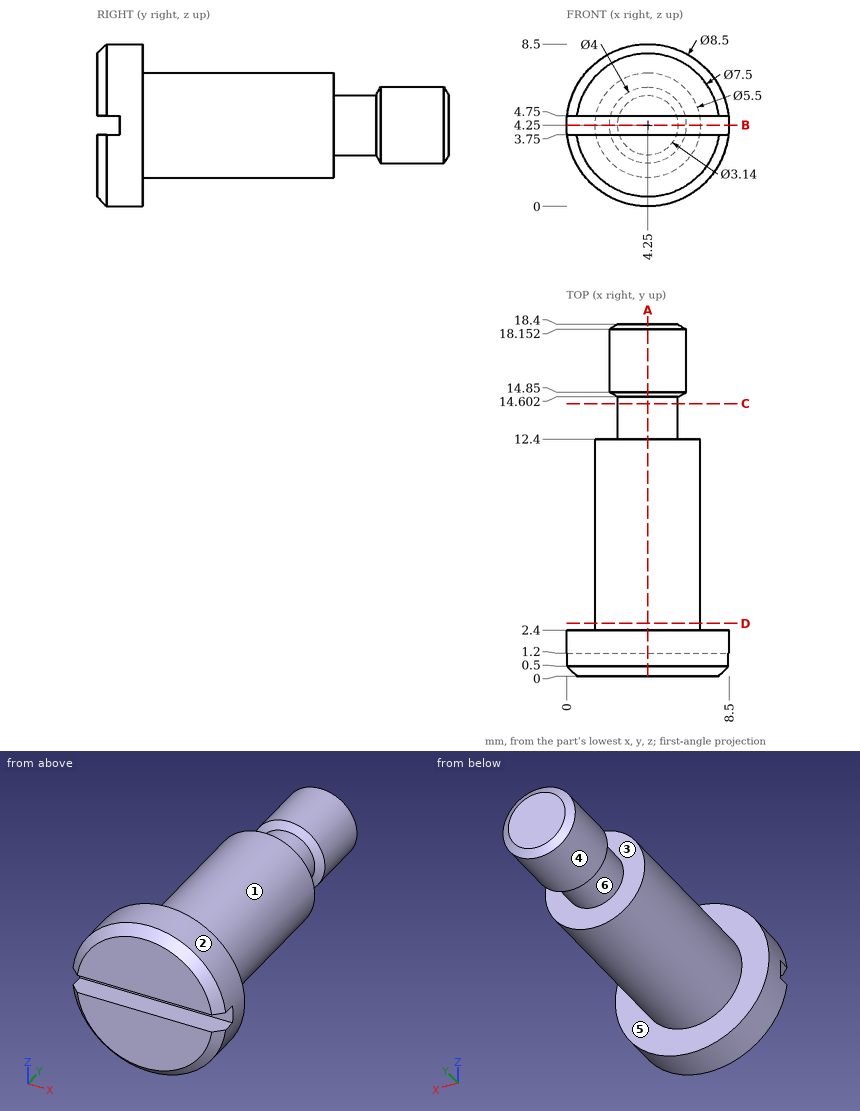
Verification items for this drawing (mm, ordinates from the low corner). A direction names the side the tool comes from. Round coordinates to 2 decimals unless told otherwise and drop trailing zeros. Loops run counter-clockwise (first coordinate to the right, second up) from the corner with the lowest first, then second, coordinate; pieces in that order, holes last. Notation, with made-up numbers: (-19, 29) -> (23, 29) arc R18 cw to (23, 38) -> close; hole circle Ø4 at (25, 33.5). An arc over 180 degrees is marked (long way). Answer in a Markdown table with one row per item.
Q1. Thickness scan on L1, parallel to Y at x = 1.75, z = 1.75; L2, parallel to Y at x = 4, z = 2; L3, parallel to Z at x = 5.25, y = 10.75. Record the ranges inside material, lowest first.
Data:
| item | result |
|---|---|
| L1 | y = 0 to 2.4 |
| L2 | y = 0 to 12.4 |
| L3 | z = 1.69 to 6.81 |
Q2. Sectioned sample at C-C on y = 14.25. Enter the section's corners in (x, z).
Data:
| item | result |
|---|---|
| outline | circle Ø3.14 at (4.25, 4.25) |
Q3. Go/stop test with flat-tipped pins: P1, Ø3, axis at x = 7, y = 14.5, coming from the -Z side; P2, Ø4, axis at x = 2.5, y = 5.5, coming from the +Z side; P3, Ø3, axis at x = 6.5, y = 14.5, coming from the +Z side. Record where each tip stops, or that it passes through.
Data:
| item | result |
|---|---|
| P1 | stops at z = 2.72 |
| P2 | stops at z = 7 |
| P3 | stops at z = 6.09 |
Q4. Sectioned sample at B-B on z = 4.25. Enter the section's corners in (x, y), then the cut area to 3 significant figures.
Data:
| item | result |
|---|---|
| outline | (0, 1.2) -> (8.5, 1.2) -> (8.5, 2.4) -> (7, 2.4) -> (7, 12.4) -> (5.82, 12.4) -> (5.82, 14.6) -> (6.25, 14.85) -> (6.25, 18.15) -> (5.82, 18.4) -> (2.68, 18.4) -> (2.25, 18.15) -> (2.25, 14.85) -> (2.68, 14.6) -> (2.68, 12.4) -> (1.5, 12.4) -> (1.5, 2.4) -> (0, 2.4) -> close |
| area | 87.1 mm^2 |
Q5. Release check for a two-part mould opening along Y. For the marked faces 3, 4, 5 and 6 record: released by +Y, released by -Y, zero draft, split by the parting line, or undercut.
Data:
| item | result |
|---|---|
| face 3 | undercut |
| face 4 | zero draft |
| face 5 | released by +Y |
| face 6 | undercut |
Q6. Sectioned sample at A-A on x = 4.25. Enter the section's corners in (y, z).
Data:
| item | result |
|---|---|
| outline | (0, 0.5) -> (0.5, 0) -> (2.4, 0) -> (2.4, 1.5) -> (12.4, 1.5) -> (12.4, 2.68) -> (14.6, 2.68) -> (14.85, 2.25) -> (18.15, 2.25) -> (18.4, 2.68) -> (18.4, 5.82) -> (18.15, 6.25) -> (14.85, 6.25) -> (14.6, 5.82) -> (12.4, 5.82) -> (12.4, 7) -> (2.4, 7) -> (2.4, 8.5) -> (0.5, 8.5) -> (0, 8) -> (0, 4.75) -> (1.2, 4.75) -> (1.2, 3.75) -> (0, 3.75) -> close |
Q7. Set-up check for the marked faces 1 and 2: record each of +Z, -Z, +X, -X, +Y, -Y from which the full face is reachable in a straight line by a thin tool's end or side.
Data:
| item | result |
|---|---|
| face 1 | +Y |
| face 2 | +Y, -Y |
Q8. Sectioned sample at D-D on y = 2.75. Enter the section's corners in (x, z).
Data:
| item | result |
|---|---|
| outline | circle Ø5.5 at (4.25, 4.25) |
